For this review, take the finished solid that the model builds, in its own axes (mm). A direction names the side the tool comes from. Give positions to 0.01 mm unless a question says otherwise; leave off trailing zeros. Loops run counter-clockwise (first coordinate to the right, second up) from the corner with the lowest first, then second, coordinate; pieces in that order, holes last. Notation, with made-up numbers: M -28,61 L 30,61 A17 cw 30,77 Z; hole C -8,67.25 d2. An arc over 180 degrees is marked long. Use CSV: the item, a comma, the result in double quotes. Start each with the question number.
1. Insertion check: P1, Ø0.8, axis at x = -68, y = 10.5, coming from the +Z side. The pin has a flat end and moves straight along its axis. Give the tip position at first contact, or say it passes through.
2. Take a section at C-C, the plane z = 2.5. Write out the cut boundary in (x, y), and give its area (3 significant figures).
3. To check wall thickness, follow line 1 (Y direction, x = 16, z = 2.5); line 2 (X direction, y = -3, z = 2.25); line 3 (X direction, y = 30.5, z = 4.75). State the ranges of each line that lie inside material, in increasing order. Write a range as [from, to].
4. Take a section at B-B, the plane x = 27.5. Write out the cut boundary in (y, z).
5. Take a section at A-A, the plane y = 3. Write out the cut boundary in (x, z), and give its area (3 significant figures).
6. The part is to be moulded in two halves that separate along X. For faces 4 (the face through (-1, 41, 0)), 5 (the face through (100, -1, 7)), 6 (the face through (71.77, 33.8, 12.46)), say which applies: pulls with the +X half, pulls with the -X half, needs draft (parallel to the pull), parting line crosses it, or undercut.
7. Tool access review of faces 1 (the face through (-71.77, -0.42, 6.5)), 2 (the face through (-1, 60, 7)), 3 (the face through (66.07, 33, 2.88)): name each direction out of +Z, -Z, +X, -X, +Y, -Y from which nothing blocks a thin tool from reaching the whole face with its end or side.
from build123d import *

# Parameters (mm, degrees)
F0_W      = 200
F0_H      = 120
F1_DEPTH  = 15
F2_W      = 146.4
F2_H      = 70.6
F3_DEPTH  = 10
F4_R      = 5
F5_R      = 5
F6_R      = 5
F7_R      = 5
F8_R      = 5
F9_W      = 135
F9_H      = 69
F10_DEPTH = 25
F11_R     = 5
F12_R     = 5
F13_R     = 5
F14_R     = 5


with BuildPart() as f1:
    # F0 (on Top) → F1 (new body)
    with BuildSketch(Plane.XY):
        Rectangle(F0_W, F0_H)
    extrude(amount=F1_DEPTH)

    # F2 (on face) → F3 (cut)
    with BuildSketch(Plane.XY.offset(15)):
        Rectangle(F2_W, F2_H)
    extrude(amount=-F3_DEPTH, mode=Mode.SUBTRACT)

    # F4
    f4_edges = [f1.edges().sort_by_distance(p)[0] for p in [
        (-73.2, 35.3, 10),
    ]]
    fillet(f4_edges, radius=F4_R)

    # F5
    f5_edges = [f1.edges().sort_by_distance(p)[0] for p in [
        (-73.2, -35.3, 10),
    ]]
    fillet(f5_edges, radius=F5_R)

    # F6
    f6_edges = [f1.edges().sort_by_distance(p)[0] for p in [
        (73.2, -35.3, 10),
    ]]
    fillet(f6_edges, radius=F6_R)

    # F7
    f7_edges = [f1.edges().sort_by_distance(p)[0] for p in [
        (73.2, 35.3, 10),
    ]]
    fillet(f7_edges, radius=F7_R)

    # F8
    f8_edges = [f1.edges().sort_by_distance(p)[0] for p in [
        (73.2, 0, 5),
        (0, 35.3, 5),
        (0, -35.3, 5),
        (-73.2, 0, 5),
    ]]
    fillet(f8_edges, radius=F8_R)

    # F9 (on face) → F10 (cut)
    with BuildSketch(Plane(origin=(0, 0, 0), x_dir=(1, 0, 0), z_dir=(0, 0, -1))):
        Rectangle(F9_W, F9_H)
    extrude(amount=-F10_DEPTH, mode=Mode.SUBTRACT)

    # F11
    f11_edges = [f1.edges().sort_by_distance(p)[0] for p in [
        (67.5, -34.5, 3.643534),
    ]]
    fillet(f11_edges, radius=F11_R)

    # F12
    f12_edges = [f1.edges().sort_by_distance(p)[0] for p in [
        (67.5, 34.5, 3.643534),
    ]]
    fillet(f12_edges, radius=F12_R)

    # F13
    f13_edges = [f1.edges().sort_by_distance(p)[0] for p in [
        (-67.5, 34.5, 3.643534),
    ]]
    fillet(f13_edges, radius=F13_R)

    # F14
    f14_edges = [f1.edges().sort_by_distance(p)[0] for p in [
        (-67.5, -34.5, 3.643534),
    ]]
    fillet(f14_edges, radius=F14_R)


solid = f1.part
Result set:
1,P1,"z = 5"
2,outline,"M -100,-60 L 100,-60 L 100,60 L -100,60 Z; hole M -67.5,-29.5 A5 ccw -62.5,-34.5 L 62.5,-34.5 A5 ccw 67.5,-29.5 L 67.5,29.5 A5 ccw 62.5,34.5 L -62.5,34.5 A5 ccw -67.5,29.5 Z"
2,area,"14,700 mm2"
3,line 1,"[-60, -34.5], [34.5, 60]"
3,line 2,"[-100, -67.5], [67.5, 100]"
3,line 3,"[-100, -67.4], [67.4, 100]"
4,outline,"M -60,0 L -34.5,0 L -34.5,7.29 A5 cw -35.3,10 L -35.3,15 L -60,15 Z; M 34.5,0 L 60,0 L 60,15 L 35.3,15 L 35.3,10 A5 cw 34.5,7.29 Z"
5,outline,"M -100,0 L -67.5,0 L -67.5,5 L -68.2,5 A5 cw -73.2,10 L -73.2,15 L -100,15 Z; M 67.5,0 L 100,0 L 100,15 L 73.2,15 L 73.2,10 A5 cw 68.2,5 L 67.5,5 Z"
5,area,"872 mm2"
6,face 4,"needs draft"
6,face 5,"pulls with the +X half"
6,face 6,"undercut"
7,face 1,"+Z"
7,face 2,"+Z, -Z, +X, -X, +Y"
7,face 3,"+Z, -Z"
